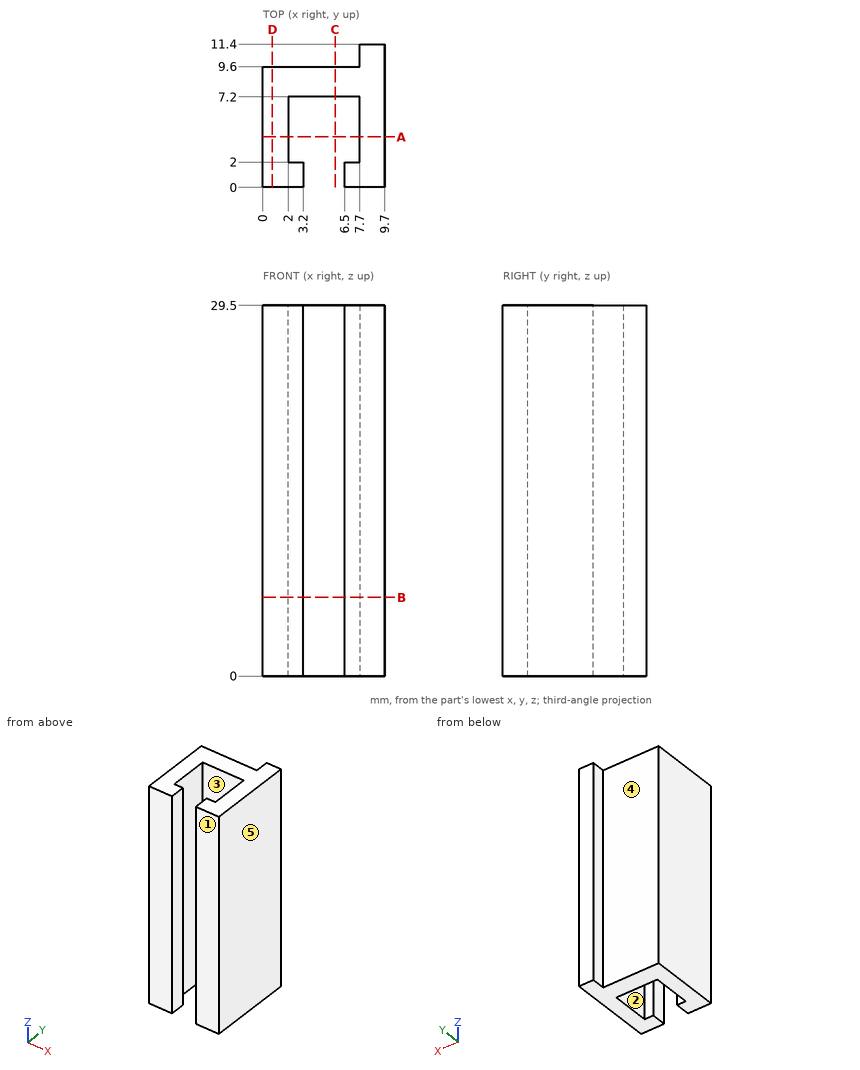
Answer from the drawing. Dimensions are ordinates in mm from the lowest x, y and z of the part. A direction names the side the tool comes from. Give positions to 0.01 mm unless a question says otherwise; leave off trailing zeros. Write each loop counter-clockwise with the first axis right and the second up, starting at its lowest first coordinate (ties: lowest second). Pieces come first, ordered by that corner, then holes. Notation, with made-up numbers: (-26, 54) - (4, 54) arc R20 cw to (4, 81) - close; hole circle Ø6 at (-20, -1). An arc over 180 degrees is marked (long way). Answer in a Markdown table with one row per item. Add a question column.
Item 1: Find the intervals of material crossed by L1, parallel to X at y = 7, z = 24; L2, parallel to Y at x = 2.5, z = 27; L3, parallel to Y at x = 4.25, z = 23.25, in increasing order.
Item 2: Section A-A, the plane y = 4 is taken. Write down the section's boundary in (x, z), and give its area (3 significant figures).
Item 3: Determine the mould class of the marked faces 3, 4 and 5 for opening direction X: pulls with the +X half, pulls with the -X half, needs draft (parallel to the pull), parting line crosses it, or undercut.
Item 4: Section D-D, the plane x = 0.75 is taken. Write down the section's boundary in (y, z), and give its area (3 significant figures).
Item 5: Flat-ended cylindrical pins translate along their axes: P1, Ø1.5, axis at x = 5.5, z = 8.5, coming from the -Y side; P2, Ø1.4, axis at y = 10.5, z = 17, coming from the -X side; P3, Ø0.6, axis at x = 2.5, z = 11.5, coming from the +Y side. Find the tip coordinate at first contact, or state that the pin passes through.
Item 6: A tool of negligible diameter and unlimited length cuts with its end or side. For the marked faces 1 and 2, from which of +Z, -Z, +X, -X, +Y, -Y can it reach the whole face along a straight path? Write none if from no direction.
Item 7: Section C-C, the plane x = 5.75 is taken. Write down the section's boundary in (y, z), and give its area (3 significant figures).
Item 8: Section B-B, the plane z = 6.25 is taken. Write down the section's boundary in (x, y).
Recorded:
| question | item | result |
|---|---|---|
| 1 | L1 | x = 0 to 2, 7.7 to 9.7 |
| 1 | L2 | y = 0 to 2, 7.2 to 9.6 |
| 1 | L3 | y = 7.2 to 9.6 |
| 2 | outline | (0, 0) - (2, 0) - (2, 29.5) - (0, 29.5) - close; (7.7, 0) - (9.7, 0) - (9.7, 29.5) - (7.7, 29.5) - close |
| 2 | area | 118 mm2 |
| 3 | face 3 | undercut |
| 3 | face 4 | needs draft |
| 3 | face 5 | pulls with the +X half |
| 4 | outline | (0, 0) - (9.6, 0) - (9.6, 29.5) - (0, 29.5) - close |
| 4 | area | 283 mm2 |
| 5 | P1 | stops at y = 7.2 |
| 5 | P2 | stops at x = 7.7 |
| 5 | P3 | stops at y = 9.6 |
| 6 | face 1 | +Z, -Z, +X, -X, -Y |
| 6 | face 2 | +Z, -Z |
| 7 | outline | (7.2, 0) - (9.6, 0) - (9.6, 29.5) - (7.2, 29.5) - close |
| 7 | area | 70.8 mm2 |
| 8 | outline | (0, 0) - (3.2, 0) - (3.2, 2) - (2, 2) - (2, 7.2) - (7.7, 7.2) - (7.7, 2) - (6.5, 2) - (6.5, 0) - (9.7, 0) - (9.7, 11.4) - (7.7, 11.4) - (7.7, 9.6) - (0, 9.6) - close |
